Here's how the part is built. I have some questions about the finished solid (model axes, mm). Face numbers are marked on the shaded views. A direction names the side the tool comes from. Round coordinates to 2 decimals unless told otherwise and drop trailing zeros. Write each loop counter-clockwise with the first axis right and the second up, starting at its lowest first coordinate (ties: lowest second). Pieces come first, ordered by that corner, then holes. Notation, with made-up numbers: (70, -6.5) - (107, -6.5) arc R26 cw to (107, 14.5) - close; hole circle Ø3 at (24.5, -22). An arc over 180 degrees is marked (long way). Use one line per item in the form item = value. Start each with the question number.
1. I want a section at D-D, the plane x = -5.5. List the corners of the cut face in (y, z) for me.
2. I want a section at B-B, the plane z = 0. List the corners of the cut face in (x, y) for me, plus the area to 3 significant figures.
3. If I drill on line 1 along Y through (x, z) = (3, -6); line 2 along Y through (x, z) = (7.25, 1.75); line 3 along Z through (x, y) = (-3, 14), over which ranges is the centre line in solid material (lowest first)?
4. Which directions (+Z, -Z, +X, -X, +Y, -Y) give clear straight access to the entire face, cutting with the end or side of a thin tool? Please do the marked faces 1, 2 and 3.
5. I want a section at A-A, the plane x = 0. List the corners of the cut face in (y, z) for me, plus the area to 3 significant figures.
6. We'd pull the mould along X, two halves only. Please class the marked faces 4, 5, 6 and 7: +X half, -X half, draft (parallel to the pull), parting line (faces both ways), or undercut.
7. I want a section at C-C, the plane y = 18.5. List the corners of the cut face in (x, z) for me.
8. Will these pins go through, and if not, where does the flat tip stop? pin 1 (4 mm diameter, centred on x = -0.5, z = 1, fed in from +Y); pin 2 (1.6 mm diameter, centred on y = 32.5, z = 0.5, fed in from -X); pin 3 (4 mm diameter, centred on x = 2.5, y = 22.5, fed in from +Z).
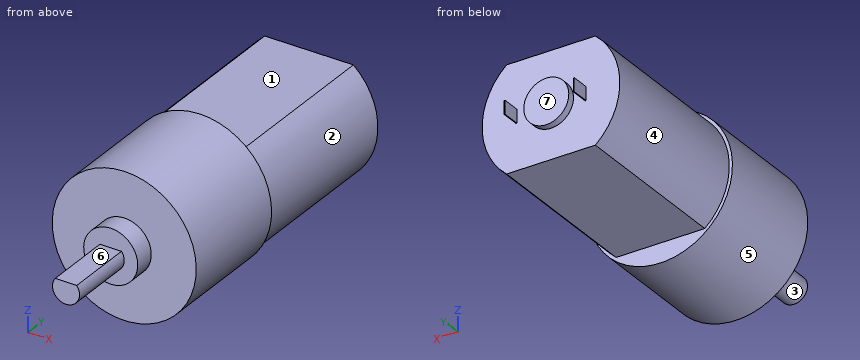
```python
from build123d import *

# Parameters (mm, degrees)
SKETCH_1_R      = 8
EXTRUDE_1_DEPTH = 12.8
EXTRUDE_2_DEPTH = 18.6
SKETCH_3_R      = 2.5
EXTRUDE_3_DEPTH = 0.8
SKETCH_4_W      = 0.091344541
SKETCH_4_H      = 1.5
EXTRUDE_4_DEPTH = 2
SKETCH_5_R      = 3
EXTRUDE_5_DEPTH = 2.3
EXTRUDE_6_DEPTH = 7.6


with BuildPart() as part:
    # Эскиз1 → Бобышка-Вытянуть1 (new body)
    with BuildSketch(Plane(origin=(0, 0, 0), x_dir=(1, 0, 0), z_dir=(0, 1, 0))):
        with Locations(Location((0, 0, 0), (0, 0, 270))):
            Circle(SKETCH_1_R)
    extrude(amount=EXTRUDE_1_DEPTH)

    # Эскиз2 → Бобышка-Вытянуть2 (add)
    with BuildSketch(Plane(origin=(0, 12.8, 0), x_dir=(1, 0, 0), z_dir=(0, 1, 0))):
        with BuildLine():
            Line((-4.929503018, 5.85), (4.929503018, 5.85))
            ThreePointArc((4.929503018, 5.85), (7.65, 0), (4.929503018, -5.85))
            Line((4.929503018, -5.85), (-4.929503018, -5.85))
            ThreePointArc((-4.929503018, -5.85), (-7.65, 0), (-4.929503018, 5.85))
        make_face()
    extrude(amount=EXTRUDE_2_DEPTH)

    # Эскиз3 → Бобышка-Вытянуть3 (add)
    with BuildSketch(Plane(origin=(0, 31.4, 0), x_dir=(1, 0, 0), z_dir=(0, 1, 0))):
        with Locations(Location((0, 0, 0), (0, 0, 270))):
            Circle(SKETCH_3_R)
    extrude(amount=EXTRUDE_3_DEPTH)

    # Эскиз4 → Бобышка-Вытянуть4 (add)
    with BuildSketch(Plane(origin=(0, 31.4, 0), x_dir=(1, 0, 0), z_dir=(0, 1, 0))):
        with Locations((-3.845672271, 0)):
            Rectangle(SKETCH_4_W, SKETCH_4_H)
        with Locations((3.845672271, 0)):
            Rectangle(SKETCH_4_W, SKETCH_4_H)
    extrude(amount=EXTRUDE_4_DEPTH)

    # Эскиз5 → Бобышка-Вытянуть5 (add)
    with BuildSketch(Plane.XZ):
        with Locations(Location((0, 0, 0), (0, 0, 90))):
            Circle(SKETCH_5_R)
    extrude(amount=EXTRUDE_5_DEPTH)

    # Эскиз6 → Бобышка-Вытянуть6 (add)
    with BuildSketch(Plane.XZ.offset(2.3)):
        with BuildLine():
            Line((-1.2, 0.9), (1.2, 0.9))
            ThreePointArc((1.2, 0.9), (0, -1.5), (-1.2, 0.9))
        make_face()
    extrude(amount=EXTRUDE_6_DEPTH)


solid = part.part
```
Model answer:
q1.outline = (0, -5.81) - (12.8, -5.81) - (12.8, -5.32) - (31.4, -5.32) - (31.4, 5.32) - (12.8, 5.32) - (12.8, 5.81) - (0, 5.81) - close
q2.outline = (-8, 0) - (-3, 0) - (-3, -2.3) - (-1.5, -2.3) - (-1.5, -9.9) - (1.5, -9.9) - (1.5, -2.3) - (3, -2.3) - (3, 0) - (8, 0) - (8, 12.8) - (7.65, 12.8) - (7.65, 31.4) - (3.89, 31.4) - (3.89, 33.4) - (3.8, 33.4) - (3.8, 31.4) - (2.5, 31.4) - (2.5, 32.2) - (-2.5, 32.2) - (-2.5, 31.4) - (-3.8, 31.4) - (-3.8, 33.4) - (-3.89, 33.4) - (-3.89, 31.4) - (-7.65, 31.4) - (-7.65, 12.8) - (-8, 12.8) - close
q2.area = 530 mm2
q3.line_1 = 0 to 12.8
q3.line_2 = 0 to 31.4
q3.line_3 = -5.85 to 5.85
q4.face_1 = +Z, +X, -X, +Y
q4.face_2 = +X, +Y
q4.face_3 = -Y
q5.outline = (-9.9, -1.5) - (-2.3, -1.5) - (-2.3, -3) - (0, -3) - (0, -8) - (12.8, -8) - (12.8, -5.85) - (31.4, -5.85) - (31.4, -2.5) - (32.2, -2.5) - (32.2, 2.5) - (31.4, 2.5) - (31.4, 5.85) - (12.8, 5.85) - (12.8, 8) - (0, 8) - (0, 3) - (-2.3, 3) - (-2.3, 0.9) - (-9.9, 0.9) - close
q5.area = 458 mm2
q6.face_4 = -X half
q6.face_5 = parting line
q6.face_6 = draft
q6.face_7 = undercut
q7.outline = (-4.93, -5.85) - (4.93, -5.85) arc R7.65 ccw to (4.93, 5.85) - (-4.93, 5.85) arc R7.65 ccw to start
q8.pin_1 = 32.2
q8.pin_2 = -3.89
q8.pin_3 = 5.85
